Autodesk Inventor part; units mm, degrees
sketch "Sketch1" plane through (0, 0, 0) normal (0, 0, 1) x (1, 0, 0)
  line L0 (-22.5, 20) -> (22.5, 20)
  line L1 (22.5, 20) -> (22.5, 0)
  line L2 (22.5, 0) -> (-22.5, 0)
  line L3 (-22.5, 0) -> (-22.5, 20)
  line L4 (-22.5, 20) -> (22.5, 0) construction
  line L5 (22.5, 20) -> (-22.5, 0) construction
  circle A0 centre (-20.4468, 18.2798) radius 1
  circle A1 centre (20.5532, 18.2798) radius 1
  circle A2 centre (20.5532, 1.7798) radius 1
  circle A3 centre (-20.4468, 1.7798) radius 1
  circle A4 centre (-12.9468, 10.0298) radius 8.2
  circle A5 centre (13.0532, 10.0298) radius 8.2
  line L6 (-3.1968, 19.7798) -> (3.3032, 19.7798)
  line L7 (-3.1968, 15.7798) -> (3.3032, 15.7798)
  arc A6 (-3.1968, 19.7798) -> (-3.1968, 15.7798) centre (-3.1968, 17.7798) ccw
  arc A7 (3.3032, 15.7798) -> (3.3032, 19.7798) centre (3.3032, 17.7798) ccw
  line L8 (-22.5, 0) -> (22.5, 0)
  line L9 (22.5, 0) -> (22.5, -20)
  line L10 (22.5, -20) -> (-22.5, -20)
  line L11 (-22.5, -20) -> (-22.5, 0)
  line L12 (-22.5, 0) -> (22.5, -20) construction
  line L13 (22.5, 0) -> (-22.5, -20) construction
  circle A8 centre (13.0532, -10) radius 2.5
  circle A9 centre (-12.9468, -10) radius 2.5
  circle A10 centre (-20.4468, 18.2798) radius 1
  circle A11 centre (-20.4468, 1.7798) radius 1
  circle A12 centre (20.5532, 18.2798) radius 1
  circle A13 centre (20.5532, 1.7798) radius 1
  line L14 (-22.5, 22) -> (22.5, 22)
  line L15 (22.5, 22) -> (22.5, 20)
  line L16 (22.5, 20) -> (-22.5, 20)
  line L17 (-22.5, 20) -> (-22.5, 22)
  point P0 (0, 0)
  point P1 (0, 10)
  point P2 (-5.1968, 17.7798)
  point P3 (0, 0)
  point P4 (5.3032, 17.7798)
  point P5 (0, -10)
  point P6 (-22.5, 0)
  point P7 (0, 20)
  dimension "d0" = 45
  dimension "d1" = 20
  dimension "d16" = 16.4
  dimension "d18" = 12.9468
  dimension "d19" = 9.9702
  dimension "d20" = 9.9702
  dimension "d21" = 13.0532
  dimension "d23" = 10.5
  dimension "d24" = 2
  dimension "d25" = 5
  dimension "d26" = 20
  dimension "d27" = 2
extrude "Extrusion2" add sketch "Sketch1" along normal mid plane 2
properties part number "suporte_ultrassonico_001_3DPrint"
The model under review builds one solid part; all positions refer to its coordinate system, in mm. A direction names the side the tool comes from. Coordinates: 2 decimals unless noted, no trailing zeros. Write each loop counter-clockwise with the first axis right and the second up, starting at its lowest first coordinate (ties: lowest second). Pieces come first, ordered by that corner, then holes. Notation, with made-up numbers: (53.5, -22) - (101.5, -22) arc R18 ccw to (101.5, -18) - close; hole circle Ø6 at (2, -4.5). An arc over 180 degrees is marked (long way). Answer in a Markdown table with one row per item. Add a question column.
Q1. Draft analysis for pull direction X (two halves, no side actions). For faces 1 (the face through (14.207, -7.782, -0.014)), 2 (the face through (-22.5, 1, 0)), 3 (the face through (0, 1, 1)), state which applies: +X half, -X half, draft (parallel to the pull), parting line (faces both ways), or undercut.
Q2. Consider section D-D on x = 15. Give the boundary of the cut face in (y, z).
Q3. Consider section A-A on y = -10. Give the boundary of the cut face in (x, z), then the cut area to 3 significant figures.
Q4. For faces 4 (the face through (0, 15.78, 0)), 5 (the face through (0, 22, 0)), list the 3-axis set-ups (+Z, -Z, +X, -X, +Y, -Y) from which the entire face can be reached by the end or side of a thin tool; tool diameter is ignored.
Q5. Consider section B-B on z = -0.5. Give the number of separate pieces and of enclosed holes in the cut face, then the cut area to 3 significant figures.
Q6. Clearance check with flat-ended pins moving along their axes: pin 1 (1.6 mm diameter, centred on x = 20.55, y = 1.78, fed in from -Z); pin 2 (8 mm diameter, centred on x = 13.05, y = -10, fed in from -Z). State where each tip first meets the part, or that it passes through.
Q7. To check wall thickness, follow line 1 along Y through (x, z) = (1.5, -0.1); line 2 along Y through (x, z) = (20, -0.9); line 3 along Y through (x, z) = (-11, 0.45). State the ranges of each line that lie inside material, in increasing order. Write a range as from..to.
Q8. Consider section C-C on x = 7. Give the boundary of the cut face in (y, z), then the cut area to 3 significant figures.
Answers below:
| question | item | result |
|---|---|---|
| 1 | face 1 | undercut |
| 1 | face 2 | -X half |
| 1 | face 3 | draft |
| 2 | outline | (-20, -1) - (-11.57, -1) - (-11.57, 1) - (-20, 1) - close; (-8.43, -1) - (2.06, -1) - (2.06, 1) - (-8.43, 1) - close; (18, -1) - (22, -1) - (22, 1) - (18, 1) - close |
| 3 | outline | (-22.5, -1) - (-15.45, -1) - (-15.45, 1) - (-22.5, 1) - close; (-10.45, -1) - (10.55, -1) - (10.55, 1) - (-10.45, 1) - close; (15.55, -1) - (22.5, -1) - (22.5, 1) - (15.55, 1) - close |
| 3 | area | 70.0 mm² |
| 4 | face 4 | +Z, -Z |
| 4 | face 5 | +Z, -Z, +X, -X, +Y |
| 5 | separate pieces | 1 |
| 5 | enclosed holes | 9 |
| 5 | area | 1,380 mm² |
| 6 | pin 1 | through |
| 6 | pin 2 | z = -1 |
| 7 | line 1 | -20..15.78, 19.78..22 |
| 7 | line 2 | -20..0.95, 2.61..5.67, 14.39..17.45, 19.11..22 |
| 7 | line 3 | -20..-11.57, -8.43..2.06, 18..22 |
| 8 | outline | (-20, -1) - (4.5, -1) - (4.5, 1) - (-20, 1) - close; (15.56, -1) - (22, -1) - (22, 1) - (15.56, 1) - close |
| 8 | area | 61.9 mm² |
